```python
from build123d import *

# Parameters (mm, degrees)
BOSS_EXTRU_1_DEPTH           = 6.5
R_P_TITION_CIRCULAIRE1_COUNT = 11
ENL_V_MAT_EXTRU_1_REACH      = 13.822


with BuildPart() as part:
    # Esquisse1 → Boss.-Extru.1 (new body)
    with BuildSketch(Plane.XY):
        with BuildLine():
            Line((2.665741612, 4.429754131), (0, 0))
            Line((0, 0), (-1.27495348, 5.010328694))
            ThreePointArc((-1.27495348, 5.010328694), (-1.158589319, 5.038508786), (-1.041603805, 5.063986721))
            ThreePointArc((-1.041603805, 5.063986721), (-0.853375021, 5.171115564), (-0.764222128, 5.368494453))
            ThreePointArc((-0.764222128, 5.368494453), (-0.587161287, 6.209477662), (-0.25, 7))
            Line((-0.25, 7), (0.25, 7))
            ThreePointArc((0.25, 7), (0.587161287, 6.209477662), (0.764222128, 5.368494453))
            ThreePointArc((0.764222128, 5.368494453), (0.853375021, 5.171115564), (1.041603805, 5.063986721))
            ThreePointArc((1.041603805, 5.063986721), (1.880602365, 4.815831677), (2.665741612, 4.429754131))
        make_face()
    boss_extru_1 = extrude(amount=BOSS_EXTRU_1_DEPTH)

    # R_p_tition circulaire1: Boss.-Extru.1 ×11 about axis
    r_p_tition_circulaire1_axis = Axis((0, 0, 0), (0, 0, 1))
    for i in range(1, R_P_TITION_CIRCULAIRE1_COUNT):
        add(boss_extru_1.rotate(r_p_tition_circulaire1_axis, i * 360 / R_P_TITION_CIRCULAIRE1_COUNT))

    # Esquisse2 → Enl_v. mat.-Extru.1 (cut, up to next)
    with BuildSketch(Plane.XY.offset(6.5), mode=Mode.PRIVATE) as enl_v_mat_extru_1_sk1:
        with BuildLine():
            Line((-2.174856317, 1.6), (2.174856317, 1.6))
            ThreePointArc((2.174856317, 1.6), (2.7, 0), (2.174856317, -1.6))
            Line((2.174856317, -1.6), (-2.174856317, -1.6))
            ThreePointArc((-2.174856317, -1.6), (-2.7, 0), (-2.174856317, 1.6))
        make_face()
    enl_v_mat_extru_1_tool1 = extrude(enl_v_mat_extru_1_sk1.sketch, amount=-ENL_V_MAT_EXTRU_1_REACH, mode=Mode.PRIVATE) & part.part
    add(enl_v_mat_extru_1_tool1.solids().sort_by_distance((0, 0, 6.5))[0], mode=Mode.SUBTRACT)


solid = part.part
```
CAD build for the part. Positions are in the model's coordinates, mm. A direction names the side the tool comes from. Round coordinates to 2 decimals unless told otherwise and drop trailing zeros. Loops run counter-clockwise (first coordinate to the right, second up) from the corner with the lowest first, then second, coordinate; pieces in that order, holes last. Notation, with made-up numbers: M 1.25,73 L 14.25,73 A8 cw 14.25,84 Z; hole C 82,27.5 d11. An arc over 180 degrees is marked long. Return JSON: item names as keys, results as strings. Group by question number.
(1) Drop flat-ended pins along their axis: P1, Ø2, axis at x = 1, z = 3.5, coming from the -Y side; P2, Ø2, axis at y = 0.5, z = 1, coming from the +X side; P3, Ø1.5, axis at y = 3.5, z = 4, coming from the -X side; P4, Ø2, axis at x = 3, z = 5, coming from the -Y side. Give the stop position or say it passes through.
(2) Saw through at D-D, the plane y = 4.5. List the corners of the cut face in (x, z).
(3) Saw through at C-C, the plane y = -3.5. List the corners of the cut face in (x, z).
(4) Tool access for faces 1 (the cylindrical face through (-3.848, 4.895, 3.204)), 2 (the cylindrical face through (-1.179, -6.113, 3.204)), 3 (the cylindrical face through (-2.872, 5.549, 3.204)): list every direction of +Z, -Z, +X, -X, +Y, -Y with a clear straight run to the whole face (end or side of a thin tool).
(5) Saw through at B-B, the plane x = -1.5. List the corners of the cut face in (y, z).
(6) Mould opens along Y. For faces 4 (the flat face through (0, 2, 0)), 5 (the flat face through (0, -1.6, 3)), 6 (the cylindrical face through (0.584, 6.221, 3.204)) say: +Y half, -Y half, draft (parallel to the pull), parting line (faces both ways), or undercut.
(7) Saw through at A-A, the plane x = 6. List the corners of the cut face in (y, z).
(8) Wall check: probe 1 along Y at (x, z) = (0, 3.5); probe 2 along X at (y, z) = (5.25, 2.75); probe 3 along X at (y, z) = (5.5, 3.75). Give the ranges that are in metal, low to high. Write a range as [from, to].
Answer list:
{
 "1": {"P1": "y = -6.79", "P2": "x = 6.6", "P3": "x = -6.44", "P4": "y = -6.71"},
 "2": {"outline": "M -3.72,0 L 3.72,0 L 3.72,6.5 L -3.72,6.5 Z"},
 "3": {"outline": "M -5,0 L 5,0 L 5,6.5 L -5,6.5 Z"},
 "4": {"face 1": "+Z, -Z, -X", "face 2": "+Z, -Z, -Y", "face 3": "+Z, -Z, +Y"},
 "5": {"outline": "M -6.54,0 L -1.6,0 L -1.6,6.5 L -6.54,6.5 Z; M 1.6,0 L 4.95,0 L 4.95,6.5 L 1.6,6.5 Z"},
 "6": {"face 4": "draft", "face 5": "undercut", "face 6": "+Y half"},
 "7": {"outline": "M -1.47,0 L -0.2,0 L -0.2,6.5 L -1.47,6.5 Z; M 2.15,0 L 3.15,0 L 3.15,6.5 L 2.15,6.5 Z"},
 "8": {"probe 1": "[-5.17, -1.6], [1.6, 7]", "probe 2": "[-3.93, -2.55], [-0.8, 0.8], [2.55, 3.93]", "probe 3": "[-3.97, -2.81], [-0.75, 0.75], [2.81, 3.97]"}
}
